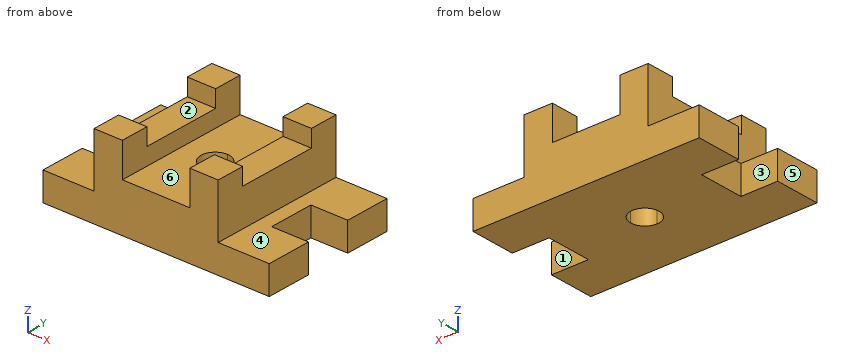
```python
from build123d import *

# Parameters (mm, degrees)
F1_DEPTH = 31.75
F0_W     = 31.75
F0_H     = 31.75
F2_DEPTH = 92.075
F0_H_2   = 88.9
F3_DEPTH = 73.025
F4_DEPTH = 53.975
F5_SCALE = 0.5


with BuildPart() as f1:
    # F0 (on Top) → F1 (new body)
    with BuildSketch(Plane.XY):
        Polygon((126.6564279795, 76.0030429602), (69.5064279795, 76.0030429602), (69.5064279795, 44.2530429602), (69.5064279795, -44.6469570398), (69.5064279795, -76.3969570398), (126.6564279795, -76.3969570398), (126.6564279795, -25.5969570398), (85.3814279795, -25.5969570398), (85.3814279795, 25.2030429602), (126.6564279795, 25.2030429602), align=None)
    extrude(amount=F1_DEPTH)

    # F0 (on Top) → F2 (join)
    with BuildSketch(Plane.XY):
        with Locations((53.6314279795, 60.1280429602)):
            Rectangle(F0_W, F0_H)
        with Locations((53.6314279795, -60.5219570398)):
            Rectangle(F0_W, F0_H)
    extrude(amount=F2_DEPTH)

    # F0 (on Top) → F3 (join)
    with BuildSketch(Plane.XY):
        with Locations((53.6314279795, -0.1969570398)):
            Rectangle(F0_W, F0_H_2)
    extrude(amount=F3_DEPTH)



with BuildPart() as f1b:
    # F0 (on Top) → F1, piece 2 (new body)
    with BuildSketch(Plane.XY):
        Polygon((-69.5064279795, 76.0030429602), (-126.6564279795, 76.0030429602), (-126.6564279795, 25.2030429602), (-85.3814279795, 25.2030429602), (-85.3814279795, -25.5969570398), (-126.6564279795, -25.5969570398), (-126.6564279795, -76.3969570398), (-69.5064279795, -76.3969570398), (-69.5064279795, -44.6469570398), (-69.5064279795, 44.2530429602), align=None)
    extrude(amount=F1_DEPTH)

    # F0 (on Top) → F2, piece 2 (join)
    with BuildSketch(Plane.XY):
        with Locations((-53.6314279795, 60.1280429602)):
            Rectangle(F0_W, F0_H)
        with Locations((-53.6314279795, -60.5219570398)):
            Rectangle(F0_W, F0_H)
    extrude(amount=F2_DEPTH)

    # F0 (on Top) → F3, piece 2 (join)
    with BuildSketch(Plane.XY):
        with Locations((-53.6314279795, -0.1969570398)):
            Rectangle(F0_W, F0_H_2)
    extrude(amount=F3_DEPTH)


with BuildPart() as f1_1:
    add(f1.part)

    add(f1b.part)  # F4 merges F1b
    # F0 (on Top) → F4 (join)
    with BuildSketch(Plane.XY):
        with BuildLine():
            Line((37.7564279795, 76.0030429602), (0, 76.0030429602))
            Line((0, 76.0030429602), (0, 15.875))
            ThreePointArc((0, 15.875), (11.2253201513, 11.2253201513), (15.875, 0))
            ThreePointArc((15.875, 0), (11.2253201513, -11.2253201513), (0, -15.875))
            Line((0, -15.875), (0, -76.3969570398))
            Line((0, -76.3969570398), (37.7564279795, -76.3969570398))
            Line((37.7564279795, -76.3969570398), (37.7564279795, -44.6469570398))
            Line((37.7564279795, -44.6469570398), (37.7564279795, 44.2530429602))
            Line((37.7564279795, 44.2530429602), (37.7564279795, 76.0030429602))
        make_face()
        with BuildLine():
            Line((0, 76.0030429602), (-37.7564279795, 76.0030429602))
            Line((-37.7564279795, 76.0030429602), (-37.7564279795, 44.2530429602))
            Line((-37.7564279795, 44.2530429602), (-37.7564279795, -44.6469570398))
            Line((-37.7564279795, -44.6469570398), (-37.7564279795, -76.3969570398))
            Line((-37.7564279795, -76.3969570398), (0, -76.3969570398))
            Line((0, -76.3969570398), (0, -15.875))
            ThreePointArc((0, -15.875), (-15.875, 0), (0, 15.875))
            Line((0, 15.875), (0, 76.0030429602))
        make_face()
    extrude(amount=F4_DEPTH)


with BuildPart() as f1_2:
    # F5: moved
    add(f1_1.part.scale(F5_SCALE))


solid = f1_2.part
```
The model under review builds one solid part; all positions refer to its coordinate system, in mm. Face numbers are marked on the shaded views. A direction names the side the tool comes from. Give positions to 0.01 mm unless a question says otherwise; leave off trailing zeros. Write each loop counter-clockwise with the first axis right and the second up, starting at its lowest first coordinate (ties: lowest second). Pieces come first, ordered by that corner, then holes. Notation, with made-up numbers: (56.5, 75.5) - (87.5, 75.5) arc R10 cw to (87.5, 86.5) - close; hole circle Ø8 at (23, -1). An arc over 180 degrees is marked (long way). Answer in a Markdown table with one row per item. Add a question column.
1. Tool access review of the marked faces 1, 2 and 3: name each direction out of +Z, -Z, +X, -X, +Y, -Y from which nothing blocks a thin tool from reaching the whole face with its end or side.
2. We need section A-A on x = 50.5. Write out the cut boundary in (y, z) (3 decimals).
3. We need section D-D on y = 3. Write out the cut boundary in (x, z) (1 decimal).
4. We need section C-C on z = 25.5. Write out the cut boundary in (x, y) (1 decimal).
5. Wall thickness on line 1 along X through (y, z) = (-24, 36.5); line 2 along Z through (x, y) = (-27, -11.5); line 3 along Z through (x, y) = (16, -19): over which ranges is each line inside the solid? List them lowest first. Write a range as [from, to].
6. Insertion check: P1, Ø9, axis at y = -2, z = 36, coming from the -X side; P2, Ø8.5, axis at x = -52, y = 8, coming from the +Z side; P3, Ø15, axis at y = 11, z = 29, coming from the +X side; P4, Ø5, axis at x = 6, y = -22, coming from the +Z side. Each pin has a flat end and moves straight along its axis. Give the tip position at first contact, or say it passes through.
7. Draft analysis for pull direction X (two halves, no side actions). For the marked faces 4, 5 and 6, state which applies: +X half, -X half, draft (parallel to the pull), parting line (faces both ways), or undercut.
8. We need section B-B on z = 31. Write out the cut boundary in (x, y), then the cut area to 3 significant figures.
Ans:
| question | item | result |
|---|---|---|
| 1 | face 1 | +Z, -Z, +X |
| 1 | face 2 | +Z, +X, -X |
| 1 | face 3 | +Z, -Z, -X |
| 2 | outline | (-38.198, 0) - (-12.798, 0) - (-12.798, 15.875) - (-38.198, 15.875) - close; (12.602, 0) - (38.002, 0) - (38.002, 15.875) - (12.602, 15.875) - close |
| 3 | outline | (-42.7, 0) - (-7.3, 0) - (-7.3, 27) - (-18.9, 27) - (-18.9, 36.5) - (-34.8, 36.5) - (-34.8, 15.9) - (-42.7, 15.9) - close; (7.3, 0) - (42.7, 0) - (42.7, 15.9) - (34.8, 15.9) - (34.8, 36.5) - (18.9, 36.5) - (18.9, 27) - (7.3, 27) - close |
| 4 | outline | (-34.8, -38.2) - (34.8, -38.2) - (34.8, 38) - (-34.8, 38) - close; hole circle Ø15.9 at (0, 0) |
| 5 | line 1 | x = [-34.75, -18.88], [18.88, 34.75] |
| 5 | line 2 | z = [0, 36.51] |
| 5 | line 3 | z = [0, 26.99] |
| 6 | P1 | stops at x = -34.75 |
| 6 | P2 | passes through |
| 6 | P3 | stops at x = 34.75 |
| 6 | P4 | stops at z = 26.99 |
| 7 | face 4 | draft |
| 7 | face 5 | -X half |
| 7 | face 6 | undercut |
| 8 | outline | (-34.75, -38.2) - (-18.88, -38.2) - (-18.88, 38) - (-34.75, 38) - close; (18.88, -38.2) - (34.75, -38.2) - (34.75, 38) - (18.88, 38) - close |
| 8 | area | 2,420 mm^2 |
